Part print with two shaded views. Sizes in mm from the minimum x, y, z corner. Round coordinates to 2 decimals unless told otherwise and drop trailing zeros. Loops run counter-clockwise (first coordinate to the right, second up) from the corner with the lowest first, then second, coordinate; pieces in that order, holes last. Notation, with made-up numbers: M 5.25,35.5 L 25.25,35.5 A25 cw 25.25,48.5 Z; hole C 61,63.25 d8. An arc over 180 degrees is marked long. Use a Markdown table: item, result. Add a question column.
Item 1: Two-plate mould, pull along X, no slides. Class the marked faces 1 and 2: +X half, -X half, draft (parallel to the pull), parting line (faces both ways), or undercut.
Item 2: Wall check: L1, parallel to X at y = 4, z = 75; L2, parallel to X at y = 5.25, z = 21; L3, parallel to X at y = 9.6, z = 75. Give the ranges that are in metal, low to high. Write a range as from..to.
Item 3: Saw through at A-A on x = 75. Write the cut outline in (y, z), then the cut area to 3 significant figures.
Item 4: Saw through at B-B on z = 75. Write the cut outline in (x, y), then the cut area to 3 significant figures.
Item 5: Saw through at D-D on z = 44. Write the cut outline in (x, y).
Item 6: Saw through at C-C on y = 4. Write the cut outline in (x, z).
Item 7: Pin check, flat tips, straight feed: P1, Ø1.5, axis at x = 36, y = 9.5, coming from the -Z side; P2, Ø3.5, axis at x = 75, z = 129, coming from the +Y side; P3, Ø9, axis at x = 75, z = 21, coming from the +Y side. Stop position of each tip, or through.
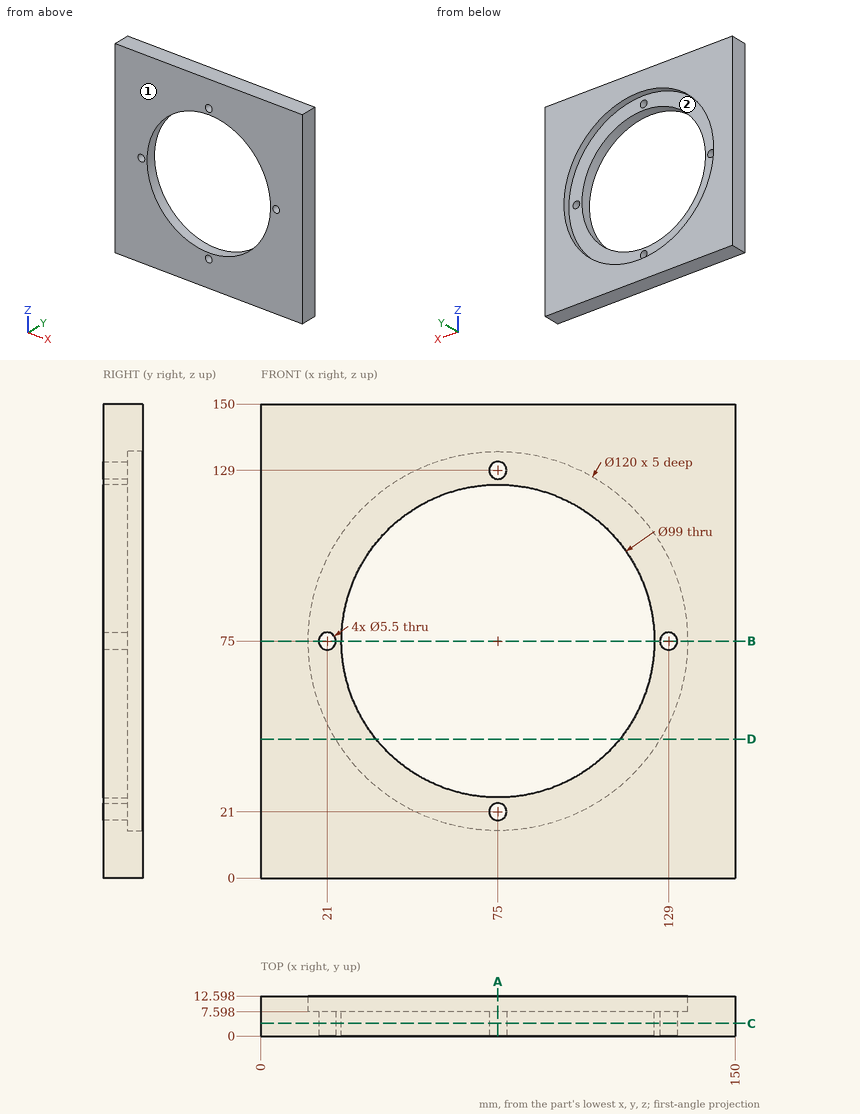
Entries:
| question | item | result |
|---|---|---|
| 1 | face 1 | draft |
| 1 | face 2 | undercut |
| 2 | L1 | 0..18.25, 23.75..25.5, 124.5..126.25, 131.75..150 |
| 2 | L2 | 0..72.25, 77.75..150 |
| 2 | L3 | 0..15, 135..150 |
| 3 | outline | M 0,0 L 12.6,0 L 12.6,15 L 7.6,15 L 7.6,18.25 L 0,18.25 Z; M 0,23.75 L 7.6,23.75 L 7.6,25.5 L 0,25.5 Z; M 0,124.5 L 7.6,124.5 L 7.6,126.25 L 0,126.25 Z; M 0,131.75 L 7.6,131.75 L 7.6,135 L 12.6,135 L 12.6,150 L 0,150 Z |
| 3 | area | 454 mm2 |
| 4 | outline | M 0,0 L 18.25,0 L 18.25,7.6 L 15,7.6 L 15,12.6 L 0,12.6 Z; M 23.75,0 L 25.5,0 L 25.5,7.6 L 23.75,7.6 Z; M 124.5,0 L 126.25,0 L 126.25,7.6 L 124.5,7.6 Z; M 131.75,0 L 150,0 L 150,12.6 L 135,12.6 L 135,7.6 L 131.75,7.6 Z |
| 4 | area | 454 mm2 |
| 5 | outline | M 0,0 L 36.41,0 L 36.41,7.6 L 23.63,7.6 L 23.63,12.6 L 0,12.6 Z; M 113.59,0 L 150,0 L 150,12.6 L 126.37,12.6 L 126.37,7.6 L 113.59,7.6 Z |
| 6 | outline | M 0,0 L 150,0 L 150,150 L 0,150 Z; hole C 21,75 d5.5; hole C 75,75 d99; hole C 75,21 d5.5; hole C 75,129 d5.5; hole C 129,75 d5.5 |
| 7 | P1 | z = 0 |
| 7 | P2 | through |
| 7 | P3 | y = 7.6 |
